from build123d import *

# Parameters (mm, degrees)
SKETCH1_R                = 21
SKETCH1_R_2              = 13.5
BOSS_EXTRUDE1_DEPTH      = 5
BOSS_EXTRUDE2_REACH      = 49.223
BOSS_EXTRUDE2_END_RADIUS = 21
SKETCH2_W                = 5
SKETCH2_H                = 42
SKETCH2_3_W              = 40
SKETCH2_3_H              = 42
SKETCH2_3_R              = 3
BOSS_EXTRUDE3_DEPTH      = 2.5
CUT_EXTRUDE4_DEPTH       = 59.566201857


with BuildPart() as part:
    # Sketch1 → Boss-Extrude1 (new body)
    with BuildSketch(Plane(origin=(0, 0, 0), x_dir=(0, 0, -1), z_dir=(1, 0, 0))):
        Circle(SKETCH1_R)
        Circle(SKETCH1_R_2, mode=Mode.SUBTRACT)
    extrude(amount=BOSS_EXTRUDE1_DEPTH)

    # Boss-Extrude2: up to this cylinder (the profile starts outside it)
    boss_extrude2_end = Plane(origin=(2.5, 0, 0), z_dir=(-1, 0, 0)) * Cylinder(BOSS_EXTRUDE2_END_RADIUS, 141.446, mode=Mode.PRIVATE)
    # Sketch2 → Boss-Extrude2 (add, up to the surface)
    with BuildSketch(Plane(origin=(0, 21, 0), x_dir=(1, 0, 0), z_dir=(0, 1, 0)), mode=Mode.PRIVATE) as boss_extrude2_sk1:
        with Locations((2.5, 0)):
            Rectangle(SKETCH2_W, SKETCH2_H)
    boss_extrude2_tool1 = extrude(boss_extrude2_sk1.sketch, amount=-BOSS_EXTRUDE2_REACH, mode=Mode.PRIVATE) - boss_extrude2_end
    add(boss_extrude2_tool1.solids().sort_by_distance((2.5, 21, 0))[0])
    add(boss_extrude2_tool1.solids().sort_by_distance((2.5, 21, 0))[1])

    # Sketch2_3 → Boss-Extrude3 (add)
    with BuildSketch(Plane(origin=(0, 21, 0), x_dir=(1, 0, 0), z_dir=(0, 1, 0))):
        with Locations((-15, 0)):
            Rectangle(SKETCH2_3_W, SKETCH2_3_H)
        with Locations(Location((-30, 0, 0), (0, 0, 270))):
            Circle(SKETCH2_3_R, mode=Mode.SUBTRACT)
    extrude(amount=BOSS_EXTRUDE3_DEPTH)

    # Sketch3 → Cut-Extrude4 (cut, through all)
    with BuildSketch(Plane.XZ.offset(-21)):
        Polygon((0, -28.471778575), (0, -21), (-35, -21), (-35, -7.216009452), (-35, 0), (-40.763754419, 0), (-40.763754419, -28.471778575), align=None)
        Polygon((-35, 21), (0, 21), (0, 27.25128432), (-40.763754419, 27.25128432), (-40.763754419, 0), (-35, 0), (-35, 7.216009452), align=None)
        Polygon((-35, -21), (0, -21), (-35, -7.216009452), align=None)
        Polygon((-35, 7.216009452), (0, 21), (-35, 21), align=None)
    extrude(amount=-CUT_EXTRUDE4_DEPTH, mode=Mode.SUBTRACT)


solid = part.part
Geometry: final body of the model. Coordinates: model frame, mm. A direction names the side the tool comes from. Round coordinates to 2 decimals unless told otherwise and drop trailing zeros. Loops run counter-clockwise (first coordinate to the right, second up) from the corner with the lowest first, then second, coordinate; pieces in that order, holes last. Notation, with made-up numbers: (-17, -31.75) - (-7, -31.75) arc R32 cw to (-7, -2.75) - close; hole circle Ø8 at (74.5, 20). An arc over 180 degrees is marked (long way). Write each question's results on one line, items separated by ' | '. Start each with the question number.
1) First-contact query: P1, Ø21, axis at y = 3, z = 4.5, coming from the -X side; P2, Ø1.5, axis at x = 0, z = 2, coming from the -Y side; P3, Ø5, axis at x = -30, z = 0, coming from the +Y side. Flat tips, straight axial feed; report the tip coordinate or a pass-through.
2) Cut plane C-C on z = -11. Return loops of the section in (x, y), then the cut area to 3 significant figures.
3) Mould query, pull axis Z, two halves, no side actions, for faces 3 (the face through (2.46, -13.18, 2.93)), 4 (the face through (2, -21, 0)), 5 (the face through (-29.1, 22.23, 2.86)), 6 (the face through (-35, 22, 0)). Classes: released by +Z, released by -Z, zero draft, split by the parting line, or undercut.
4) Cut plane B-B on y = 4. Return loops of the section in (x, z), then the cut area to 3 significant figures.
5) Cut plane A-A on z = 0. Return loops of the section in (x, y).
6) Access query for faces 1 (the face through (-11, 23.5, 0)), 2 (the face through (0, 14, 0)). Directions: +Z, -Z, +X, -X, +Y, -Y. A direction counts if a zero-diameter tool reaches every point of the face in a straight line with its end or side. Return the directions, or none.
7) Cut plane D-D on x = -30. Return loops of the section in (y, z).
8) Line query: probe 1 along Y at (x, z) = (2, 0); probe 2 along X at (y, z) = (-6, -15); probe 3 along X at (y, z) = (22.55, 0). Output: solid intervals per line, ascending. Write a range as [from, to].
Verdict:
1) P1: stops at x = 0 | P2: stops at y = -20.96 | P3: passes through
2) outline: (-25.39, 21) - (0, 21) - (0, 7.83) - (5, 7.83) - (5, 23.5) - (-25.39, 23.5) - close; (0, -17.89) - (5, -17.89) - (5, -7.83) - (0, -7.83) - close | area: 192 mm2
3) face 3: undercut | face 4: split by the parting line | face 5: undercut | face 6: zero draft
4) outline: (0, -21) - (5, -21) - (5, -12.89) - (0, -12.89) - close; (0, 12.89) - (5, 12.89) - (5, 21) - (0, 21) - close | area: 81.1 mm2
5) outline: (-35, 21) - (-33, 21) - (-33, 23.5) - (-35, 23.5) - close; (-27, 21) - (0, 21) - (0, 13.5) - (5, 13.5) - (5, 23.5) - (-27, 23.5) - close; (0, -21) - (5, -21) - (5, -13.5) - (0, -13.5) - close
6) face 1: +Z, -Z, +X, -X, +Y | face 2: +Z, -Z, -X, -Y
7) outline: (21, -9.19) - (23.5, -9.19) - (23.5, -3) - (21, -3) - close; (21, 3) - (23.5, 3) - (23.5, 9.19) - (21, 9.19) - close
8) probe 1: y = [-21, -13.5], [13.5, 23.5] | probe 2: x = [0, 5] | probe 3: x = [-35, -33], [-27, 5]
